Build history of the part. All positions in model axes, mm. A direction names the side the tool comes from. Coordinates: 2 decimals unless noted, no trailing zeros. Order: outer loops, then holes, each group sorted by start corner. A loop starts at its lowest first (then second) coordinate and runs counter-clockwise, first axis right, second up. Notation, with made-up numbers: (-24, 12.5) - (20, 12.5) arc R35 cw to (20, 47.5) - close; hole circle Ø9 at (-21, 6.25). An arc over 180 degrees is marked (long way). One line per item, written item: value.
from build123d import *

# Parameters (mm, degrees)
F0_W     = 82.5
F0_H     = 25.4
F1_DEPTH = 200
F2_W     = 82.5
F2_H     = 134
F3_DEPTH = 50.35
F4_DEPTH = 200


with BuildPart() as f1:
    # F0 (on Top) → F1 (new body)
    with BuildSketch(Plane.XY):
        Rectangle(F0_W, F0_H)
    extrude(amount=F1_DEPTH)

    # F2 (on face) → F3 (join)
    with BuildSketch(Plane.XZ.offset(12.7)):
        with Locations((0, 133)):
            Rectangle(F2_W, F2_H)
    extrude(amount=F3_DEPTH)

    # F4 (add): a face of the model
    f4_faces = [f1.faces().sort_by_distance(p)[0] for p in [
        (0, 0, 0),
    ]]
    extrude(f4_faces, amount=F4_DEPTH)


solid = f1.part
1. Band-saw the part on C-C, the plane z = -111. Give the cut face in (x, y).
Values found:
outline: (-41.25, -12.7) - (41.25, -12.7) - (41.25, 12.7) - (-41.25, 12.7) - close
2. Band-saw the part on B-B, the plane y = -49.5. Give the cut face in (x, z), and give its area (3 significant figures).
Values found:
outline: (-41.25, 66) - (41.25, 66) - (41.25, 200) - (-41.25, 200) - close
area: 11,100 mm2
3. Flat gauge pin, fed straight in: P1, Ø8, axis at x = -31.5, z = -72.5, coming from the -Y side. Where does the tip first touch, or does it go through?
Values found:
P1: stops at y = -12.7
4. 3-axis set-ups, long thin cutter, end or side, ignore diameter. For faces 1 (the face through (41.25, -9, 47)), 2 (the face through (-1, -38, 66)): which of +Z, -Z, +X, -X, +Y, -Y reach the whole face in a straight line?
Values found:
face 1: +Z, -Z, +X, +Y, -Y
face 2: -Z, +X, -X, -Y
5. Probe line 1 along Y through (x, z) = (33, -22.5); line 2 along Z through (x, y) = (8, -50). List the from-to ranges inside material, lowest first.
Values found:
line 1: y = -12.7 to 12.7
line 2: z = 66 to 200
6. Band-saw the part on A-A, the plane x = 13. Give the cut face in (y, z), and give its area (3 significant figures).
Values found:
outline: (-63.05, 66) - (-12.7, 66) - (-12.7, -200) - (12.7, -200) - (12.7, 200) - (-63.05, 200) - close
area: 16,900 mm2
